```python
from build123d import *

# Parameters (mm, degrees)
F0_W     = 76.2
F0_H     = 63.5
F1_DEPTH = 127
F2_T     = -5.08
F3_R     = 5.08


with BuildPart() as f1:
    # F0 (on Front) → F1 (new body)
    with BuildSketch(Plane.XZ):
        with Locations((38.1, 28.927778)):
            Rectangle(F0_W, F0_H)
    extrude(amount=F1_DEPTH)

    # F2
    f2_openings = [f1.faces().sort_by_distance(p)[0] for p in [
        (38.1, -127, 28.927778),
    ]]
    offset(amount=F2_T, openings=f2_openings)

    # F3
    f3_edges = [f1.edges().sort_by_distance(p)[0] for p in [
        (76.2, -63.5, 60.677778),
        (0, -63.5, 60.677778),
        (76.2, -63.5, -2.822222),
    ]]
    fillet(f3_edges, radius=F3_R)


solid = f1.part
```
Here's how the part is built. I have some questions about the finished solid (model axes, mm). A direction names the side the tool comes from. Give positions to 0.01 mm unless a question says otherwise; leave off trailing zeros. Write each loop counter-clockwise with the first axis right and the second up, starting at its lowest first coordinate (ties: lowest second). Pieces come first, ordered by that corner, then holes. Notation, with made-up numbers: (-31, 47) -> (15, 47) arc R14 ccw to (15, 60) -> close; hole circle Ø2 at (-3, 23.25). An arc over 180 degrees is marked (long way). Use one line per item in the form item = value.
1) Suppose I cut it at A-A (y = -61). Please give me the cut outline in (x, z), and give its area (3 significant figures).
Verdict:
outline = (0, -2.82) -> (71.12, -2.82) arc R5.08 ccw to (76.2, 2.26) -> (76.2, 55.6) arc R5.08 ccw to (71.12, 60.68) -> (5.08, 60.68) arc R5.08 ccw to (0, 55.6) -> close; hole (5.08, 2.26) -> (71.12, 2.26) -> (71.12, 55.6) -> (5.08, 55.6) -> close
area = 1,300 mm2
2) If I drill on L1, parallel to Z at x = 32, y = -10.5; L2, parallel to X at y = -106, z = 9; L3, parallel to Y at x = 35, z = 5, over which ranges is the centre line in solid material (lowest first)? Write a range as [from, to].
Verdict:
L1 = [-2.82, 2.26], [55.6, 60.68]
L2 = [0, 5.08], [71.12, 76.2]
L3 = [-5.08, 0]
3) I'm going to push a flat-ended pin straight in: pin 1 (3 mm diameter, centred on x = 20, z = 31.5, fed in from -Y). Where does the tip first touch, or does it pass through?
Verdict:
pin_1 = -5.08
4) On a 3-axis mill with a long thin cutter (end or side, diameter ignored), from which of +Z, -Z, +X, -X, +Y, -Y can I reach the whole of each face in a straight line? I mean faces 1 (the face through (38, -65, 55.598)), 2 (the face through (38, -63, 60.678)). Say none if no direction works.
Verdict:
face_1 = -Y
face_2 = +Z, +X, -X, +Y, -Y
5) Suppose I cut it at C-C (x = 52). Please give me the cut outline in (y, z).
Verdict:
outline = (-127, -2.82) -> (0, -2.82) -> (0, 60.68) -> (-127, 60.68) -> (-127, 55.6) -> (-5.08, 55.6) -> (-5.08, 2.26) -> (-127, 2.26) -> close
6) Suppose I cut it at B-B (z = 12). Please give me the cut outline in (x, y).
Verdict:
outline = (0, -127) -> (5.08, -127) -> (5.08, -5.08) -> (71.12, -5.08) -> (71.12, -127) -> (76.2, -127) -> (76.2, 0) -> (0, 0) -> close
7) We'd pull the mould along Z, two halves only. Please class faces 3 (the face through (5.08, -65, 29)), 4 (the face through (38, -127, 1)), 5 (the face through (74.672, -64.389, -1.374)): +Z half, -Z half, draft (parallel to the pull), parting line (faces both ways), or undercut.
Verdict:
face_3 = undercut
face_4 = draft
face_5 = -Z half
